Autodesk Inventor part; units mm, degrees
ref_plane "Work Plane1" through (-17.0058, 0, 0) normal (0, -0.866, -0.5) x (1, 0, 0)
ref_plane "YZ Plane" through (0, 0, 0) normal (1, 0, 0) x (0, 1, 0)
ref_plane "XZ Plane" through (0, 0, 0) normal (0, 1, 0) x (-1, 0, 0)
sketch "Sketch1" plane through (0, 0, 0) normal (1, 0, 0) x (0, 1, 0)
  line L0 (-9.2376, 0) -> (-4.6188, 8)
  line L1 (-4.6188, 8) -> (4.6188, 8)
  line L2 (4.6188, 8) -> (9.2376, 0)
  line L3 (9.2376, 0) -> (4.6188, -8)
  line L4 (4.6188, -8) -> (-4.6188, -8)
  line L5 (-4.6188, -8) -> (-9.2376, 0)
  point P0 (0, 0)
  point P1 (0, 0)
  dimension "d0" = 18.4752
extrude "Body" add sketch "Sketch1" along normal blind 9.3
sketch "Sketch2" plane through (0, 0, 0) normal (0, 0, 1) x (1, 0, 0)
  line L0 (0, 4.6188) -> (0, 9.2376)
  line L1 (0, 9.2376) -> (9.3, 9.2376)
  line L2 (9.3, 4.6188) -> (9.3, 9.2376)
  line L3 (-1.86, 0) -> (11.16, 0)
  line L4 (1.1187, 9.2376) -> (0, 7.3)
  line L5 (8.1813, 9.2376) -> (9.3, 7.3)
  dimension "d3" = 30
  dimension "d4" = 30
  dimension "d5" = 14.6
  dimension "d6" = 14.6
revolve "Chamfer1" cut sketch "Sketch2" angle 360 about axis through (-10, 0, 0) along (1, 0, 0)
sketch "Sketch3" plane through (9.3, 0, 0) normal (1, 0, 0) x (0, 0, -1)
  arc A0 (-0.625, -1.0825) -> (0.625, -1.0825) centre (0, 0) ccw
hole "Thread" at (9.3, 0, 0) direction (-1, 0, 0) diameter 8.376 end through all
chamfer "Chamfer2" distance 0.8119 angle 30 1 edges at (9.3, 0, 4.188) measured on face at (9.3, 6.1818, -0.7506)
chamfer "Chamfer3" distance 0.8119 angle 30 1 edges at (0, 0, 4.188) measured on face at (0, 6.1818, -0.7506)
ref_plane "Work Plane1" through (-17.0058, 0, 0) normal (0, -0.866, -0.5) x (1, 0, 0)
equation "\"d0\" = 1.1547 * SW"
equation "\"d1\" = KOH"
equation "\"d8\" = -0.5 * GD1 + 0.5 * NND"
equation "\"d40\" = -0.5 * GD1 + 0.5 * NND"
equation "\"d10\" = -0.5 * GD1 + 0.5 * NND"
equation "\"d41\" = -0.5 * GD1 + 0.5 * NND"
equation "\"d3\" = ANG1"
equation "\"d4\" = ANG2"
equation "\"d5\" = SW0"
equation "\"d6\" = SW01"
equation "\"ANG1\" = 30deg"
equation "\"ANG2\" = 30deg"
equation "\"KOH\" = 9.3"
equation "\"SW\" = 16"
equation "\"SW0\" = 14.6"
equation "\"SW01\" = SW0"
equation "\"GUL\" = 0.541266 * PTC"
equation "\"TOA\" = 30deg"
equation "\"PTC\" = 1.5"
equation "\"E0\" = 1.155 * SW"
equation "\"GAL\" = 0.541266 * PTC"
properties part number "ISO 4033 - M10" material "Steel"
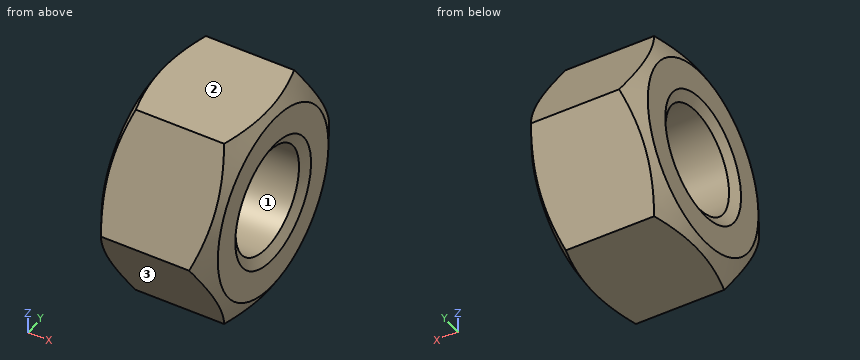
Model file for the job. Use its own axes, mm. Face numbers are marked on the shaded views. Give positions to 0.01 mm unless a question says otherwise; leave off trailing zeros. Order: outer loops, then holes, each group sorted by start corner. A loop starts at its lowest first (then second) coordinate and runs counter-clockwise, first axis right, second up.
1) Saw through at B-B, the plane y = 0. Write the cut outline in (x, z).
2) Pin check, flat tips, straight feed: pin 1 (3 mm diameter, centred on x = 6, z = -4.5, fed in from +Y); pin 2 (2 mm diameter, centred on x = 5.5, z = -6, fed in from -Y); pin 3 (4 mm diameter, centred on x = 5, z = 0.5, fed in from +Y). Stop position of each tip, or through.
3) Wall check: probe 1 along Z at (x, y) = (5, 0); probe 2 along Y at (x, z) = (5, -0.25); probe 3 along Y at (x, z) = (8.5, 3.25). Give the ranges that are in metal, low to high.
4) Mould opens along Y. For the marked faces 1, 2 and 3 say: +Y half, -Y half, draft (parallel to the pull), parting line (faces both ways), or undercut.
5) Saw through at A-A, the plane x = 7.5. Write the cut outline in (y, z), then the cut area to 3 significant figures.
Computed:
1. outline: (0, -7.3) - (0.4, -8) - (8.9, -8) - (9.3, -7.3) - (9.3, -5) - (8.83, -4.19) - (0.47, -4.19) - (0, -5) - close; (0, 5) - (0.47, 4.19) - (8.83, 4.19) - (9.3, 5) - (9.3, 7.3) - (8.9, 8) - (0.4, 8) - (0, 7.3) - close
2. pin 1: stops at y = 7.51
2. pin 2: stops at y = -6.35
2. pin 3: stops at y = 9.24
3. probe 1: z = -8 to -4.19, 4.19 to 8
3. probe 2: y = -9.09 to -4.18, 4.18 to 9.09
3. probe 3: y = -7.36 to -2.64, 2.64 to 7.36
4. face 1: undercut
4. face 2: draft
4. face 3: -Y half
5. outline: (-9.24, 0) - (-4.62, -8) - (4.62, -8) - (9.24, 0) - (4.62, 8) - (-4.62, 8) - close; hole circle Ø8.38 at (0, 0)
5. area: 167 mm2
